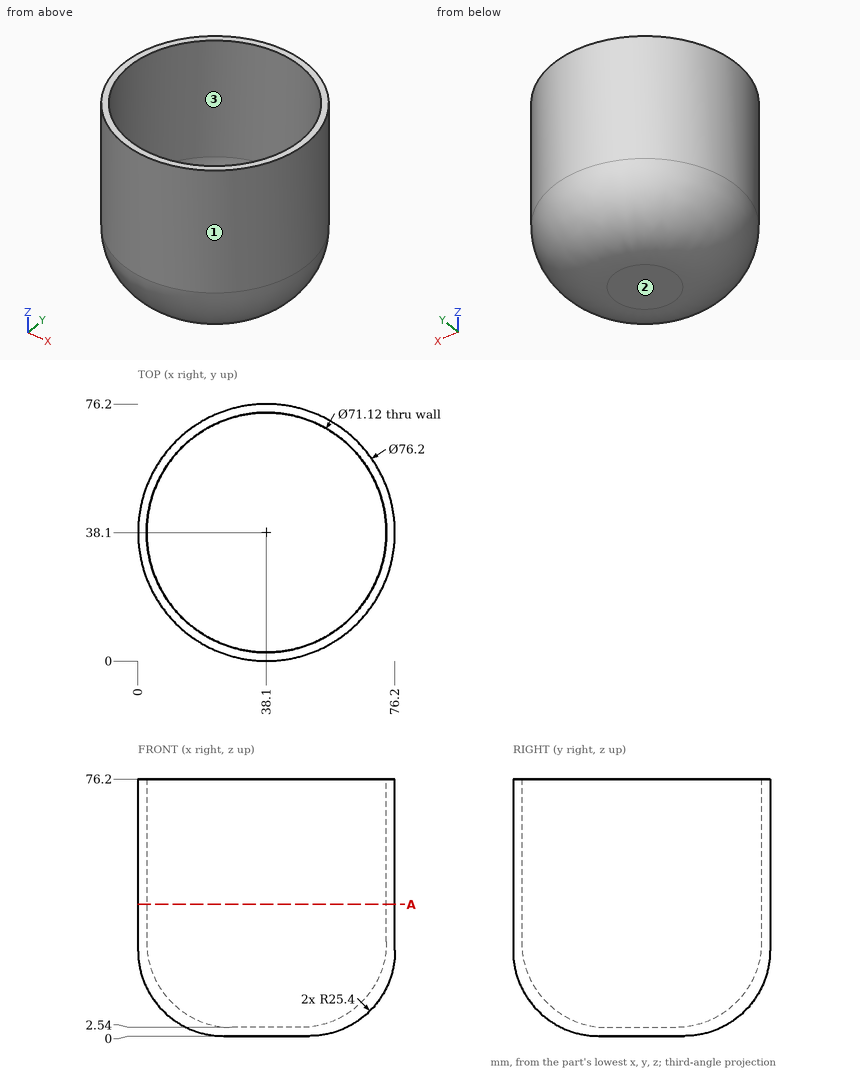
Design review of the part shown in the three views and the two pictorial views. Dimensions are in mm from the part's minimum x, y and z. Give positions to 0.01 mm unless a question says otherwise; leave off trailing zeros. Write each loop counter-clockwise with the first axis right and the second up, starting at its lowest first coordinate (ties: lowest second). Pieces come first, ordered by that corner, then holes. Notation, with made-up numbers: M -23,56.25 L -4,56.25 A8 ccw -4,70.25 Z; hole C 76.5,-5.75 d7. An arc over 180 degrees is marked long. Return JSON: item names as keys, results as strings. Group by question number.
Item 1: The part is to be moulded in two halves that separate along Y. For the marked faces 1, 2 and 3, say which applies: pulls with the +Y half, pulls with the -Y half, needs draft (parallel to the pull), parting line crosses it, or undercut.
Item 2: Clearance check with flat-ended pins moving along their axes: pin 1 Ø22.5 at (x, y) = (41, 37) entering from +Z; pin 2 Ø4 at (x, z) = (54, 60) entering from +Y; pin 3 Ø4 at (y, z) = (28, 55.5) entering from -X. State where each tip first meets the part, or that it passes through.
Item 3: Take a section at A-A (z = 39). Give the boundary of the cut face in (x, y), plus the area to 3 significant figures.
Item 4: Wall thickness on line 1 along Y through (x, z) = (38.1, 52); line 2 along Y through (x, z) = (68.5, 21.5): over which ranges is each line inside the solid? List them lowest first.
Return value:
{
 "1": {"face 1": "parting line crosses it", "face 2": "needs draft", "face 3": "undercut"},
 "2": {"pin 1": "stops at z = 2.89", "pin 2": "stops at y = 73.57", "pin 3": "stops at x = 0.87"},
 "3": {"outline": "C 38.1,38.1 d76.2; hole C 38.1,38.1 d71.12", "area": "588 mm2"},
 "4": {"line 1": "y = 0 to 2.54, 73.66 to 76.2", "line 2": "y = 15.64 to 21.31, 54.89 to 60.56"}
}
